Verification items for the finished model (mm, model axes). A direction names the side the tool comes from. Round coordinates to 2 decimals unless told otherwise and drop trailing zeros. Order: outer loops, then holes, each group sorted by start corner. A loop starts at its lowest first (then second) coordinate and runs counter-clockwise, first axis right, second up. Notation, with made-up numbers: M -20.5,35.25 L -5.5,35.25 A14 ccw -5.5,60.25 Z; hole C -0.75,63.5 d1. An arc over 180 degrees is marked long. Answer as a JSON object with one key per item and string values. Group by question number.
```python
from build123d import *

# Parameters (mm, degrees)
SKETCH_1_R          = 1.5
SKETCH_1_W          = 8
SKETCH_1_H          = 6
EXTRUDE_2_DEPTH     = 6
SKETCH_1_4_W        = 8
SKETCH_1_4_H        = 3
EXTRUDE_3_DEPTH     = 3
EXTRUDE_28_DEPTH    = 8
SKETCH_8_R          = 1.542364341
CUT_EXTRUDE_2_DEPTH = 12


with BuildPart() as part:
    # Sketch 1 → Extrude 2 (new body)
    # profile 1 of 2: a face of its own
    with BuildSketch(Plane(origin=(0, 0, 0), x_dir=(1, 0, 0), z_dir=(0, 1, 0))):
        with BuildLine():
            Line((-38.676968887, 3), (-6.676968887, 3))
            ThreePointArc((-6.676968887, 3), (-3.676968887, 0), (-6.676968887, -3))
            Line((-6.676968887, -3), (-38.676968887, -3))
            ThreePointArc((-38.676968887, -3), (-41.676968887, 0), (-38.676968887, 3))
        make_face()
        with Locations(Location((-6.676968887, 0, 0), (0, 0, 270))):
            Circle(SKETCH_1_R, mode=Mode.SUBTRACT)
        with Locations(Location((-38.676968887, 0, 0), (0, 0, 270))):
            Circle(SKETCH_1_R, mode=Mode.SUBTRACT)
    # profile 2 of 2: a face of its own
    with BuildSketch(Plane(origin=(0, 0, 0), x_dir=(1, 0, 0), z_dir=(0, 1, 0))):
        with Locations((-30.164668836, 0)):
            Rectangle(SKETCH_1_W, SKETCH_1_H)
    extrude(amount=-EXTRUDE_2_DEPTH)

    # Sketch 1_4 → Extrude 3 (add)
    with BuildSketch(Plane(origin=(0, 0, 0), x_dir=(1, 0, 0), z_dir=(0, 1, 0))):
        with Locations((-30.164668836, -1.5)):
            Rectangle(SKETCH_1_4_W, SKETCH_1_4_H)
        with Locations((-30.164668836, 1.5)):
            Rectangle(SKETCH_1_4_W, SKETCH_1_4_H)
    extrude(amount=EXTRUDE_3_DEPTH)

    # Sketch 3 → Extrude 28 (add)
    with BuildSketch(Plane(origin=(-26.164668836, 0, 0), x_dir=(0, 0, -1), z_dir=(1, 0, 0))):
        with BuildLine():
            Line((3, -2.291502622), (12.260129589, 8.208497378))
            ThreePointArc((12.260129589, 8.208497378), (11.9058809, 13.854248689), (6.260129589, 13.5))
            Line((6.260129589, 13.5), (-3, 3))
            Line((-3, 3), (3, -2.291502622))
        make_face()
    extrude(amount=-EXTRUDE_28_DEPTH)

    # Sketch 8 → Cut-Extrude 2 (cut)
    with BuildSketch(Plane(origin=(-26.164668836, 0, 0), x_dir=(0, 0, -1), z_dir=(1, 0, 0))):
        with Locations((9.921567416, 11.604248689)):
            Circle(SKETCH_8_R)
    extrude(amount=-CUT_EXTRUDE_2_DEPTH, mode=Mode.SUBTRACT)


solid = part.part
```
Q1. Cross-section at B-B, the plane z = 0. Record the cut outline in (x, y).
Q2. Cross-section at A-A, the plane x = -6. Record the cut outline in (y, z), then the cut area to 3 significant figures.
Q3. Thickness scan on line 1 (X direction, y = 3, z = -4.25); line 2 (Y direction, x = -23.5, z = 2); line 3 (Z direction, x = -22, y = -2.75). Record the ranges inside material, lowest first. Write a range as from..to.
Q4. Cross-section at C-C, the plane y = -0.5. Record the cut outline in (x, z).
Q5. Release check for a two-part mould opening along Z. For faces 1 (the face through (-3.678, -2.958, -0.066)), 2 (the face through (-22, -2, 3)), 3 (the face through (-5.19, -2.96, -0.2)) record: released by +Z, released by -Z, zero draft, split by the parting line, or undercut.
Q6. Cross-section at D-D, the plane x = -31. Record the cut outline in (y, z).
Q7. Tool access check on faces 4 (the face through (-30.109, 2.885, -7.565)), 5 (the face through (-37, 0, 0)), 6 (the face through (-15, 0, 0)). Record the directions out of +Z, -Z, +X, -X, +Y, -Y that give a thin tool (end or side, any length) a straight path to the whole face; none if there is none.
Q8. Gauge pin test, flat ends, axial feed: pin 1 Ø6.5 at (x, z) = (-17, 1) entering from +Y; pin 2 Ø5 at (y, z) = (10, -9) entering from -X; pin 3 Ø6 at (y, z) = (3, -4.5) entering from +X; pin 4 Ø1.5 at (y, z) = (9.5, -0.5) entering from +X. Record the tip position at first contact, or that the pin passes through.
Conclusion:
{
 "1": {"outline": "M -41.68,-6 L -40.18,-6 L -40.18,0 L -41.68,0 Z; M -37.18,-6 L -8.18,-6 L -8.18,0 L -26.16,0 L -26.16,6.4 L -34.16,6.4 L -34.16,0 L -37.18,0 Z; M -5.18,-6 L -3.68,-6 L -3.68,0 L -5.18,0 Z"},
 "2": {"outline": "M -6,-2.92 L 0,-2.92 L 0,-1.34 L -6,-1.34 Z; M -6,1.34 L 0,1.34 L 0,2.92 L -6,2.92 Z", "area": "19.0 mm2"},
 "3": {"line 1": "-34.16..-26.16", "line 2": "-6..0", "line 3": "-3..3"},
 "4": {"outline": "M -38.68,-3 L -34.16,-3 L -34.16,-4.58 L -26.16,-4.58 L -26.16,-3 L -6.68,-3 A3 ccw -6.68,3 L -38.68,3 A3 ccw Z; hole C -38.68,0 d3; hole C -6.68,0 d3"},
 "5": {"face 1": "split by the parting line", "face 2": "released by +Z", "face 3": "undercut"},
 "6": {"outline": "M -6,-3 L -2.29,-3 L 8.21,-12.26 A4 ccw 13.5,-6.26 L 3,3 L -6,3 Z; hole C 11.6,-9.92 d3.08"},
 "7": {"face 4": "-Z, +X, -X, -Y", "face 5": "+Z, -Z, -X, +Y", "face 6": "+Z, -Z, +X, +Y"},
 "8": {"pin 1": "y = 0", "pin 2": "x = -34.16", "pin 3": "x = -26.16", "pin 4": "through"}
}
